from build123d import *

# Parameters (mm, degrees)
EXTRUDE_1_DEPTH      = 2
SKETCH_2_W           = 7
SKETCH_2_H           = 24
SKETCH_2_W_2         = 6
SKETCH_2_H_2         = 23
EXTRUDE_2_DEPTH      = 2
SCALE_1_SCALE        = 3.5
SKETCH_4_W           = 15
SKETCH_4_H           = 100
EXTRUDE_3_DEPTH      = 100
EXTRUDE_3_DEPTH_BACK = 107
SKETCH_5_W           = 116.879299814
SKETCH_5_H           = 13.538789425
EXTRUDE_4_DEPTH      = 207
SKETCH_6_W           = 116.879299814
SKETCH_6_H           = 12
EXTRUDE_5_DEPTH      = 100
EXTRUDE_9_DEPTH      = 25
CUT_EXTRUDE_7_DEPTH  = 20
EXTRUDE_10_DEPTH     = 207
SKETCH_17_R          = 3
CUT_EXTRUDE_8_DEPTH  = 6
SKETCH_22_R          = 1.052884015
CUT_EXTRUDE_9_DEPTH  = 209.5
SKETCH_23_R          = 3.020401844
CUT_EXTRUDE_10_DEPTH = 10
SKETCH_25_R          = 1.39267654
CUT_EXTRUDE_11_DEPTH = 10


with BuildPart() as part:
    # 草图1 → 凸台-拉伸1 (new body)
    with BuildSketch(Plane.XY):
        with BuildLine():
            Line((20, -3.5), (-20, -3.5))
            ThreePointArc((-20, -3.5), (-23.5, 0), (-20, 3.5))
            Line((-20, 3.5), (20, 3.5))
            ThreePointArc((20, 3.5), (23.5, 0), (20, -3.5))
        make_face()
        with BuildLine():
            Line((20, -3), (-20, -3))
            ThreePointArc((-20, -3), (-23, 0), (-20, 3))
            Line((-20, 3), (20, 3))
            ThreePointArc((20, 3), (23, 0), (20, -3))
        make_face(mode=Mode.SUBTRACT)
    extrude(amount=EXTRUDE_1_DEPTH)

    # 草图2 → 凸台-拉伸2 (add)
    with BuildSketch(Plane.XY.offset(2)):
        with Locations((0, 15.5)):
            Rectangle(SKETCH_2_W, SKETCH_2_H)
        with Locations((0, 15.5)):
            Rectangle(SKETCH_2_W_2, SKETCH_2_H_2, mode=Mode.SUBTRACT)
    extrude(amount=-EXTRUDE_2_DEPTH)


with BuildPart() as part_1:
    # 缩放比例1: scaled about (0, 5.797269405, 1)
    add(part.part.scale(SCALE_1_SCALE).moved(Location((0, -14.493173513, -2.5))))

    # 草图4 → 凸台-拉伸3 (add, two sides)
    with BuildSketch(Plane.XY.offset(4.5)) as extrude_3_sk:
        with Locations((62.5, -76.743173512)):
            Rectangle(SKETCH_4_W, SKETCH_4_H)
        with BuildLine():
            Line((-82.25, -14.493173512), (-82.25, -126.743173512))
            Line((-82.25, -126.743173512), (-61.879299814, -126.743173512))
            Line((-61.879299814, -126.743173512), (-61.879299814, -26.743173512))
            Line((-61.879299814, -26.743173512), (-70, -26.743173512))
            ThreePointArc((-70, -26.743173512), (-78.66205807, -23.155231582), (-82.25, -14.493173512))
        make_face()
    extrude(amount=EXTRUDE_3_DEPTH)
    extrude(extrude_3_sk.sketch, amount=-EXTRUDE_3_DEPTH_BACK)

    # 草图5 → 凸台-拉伸4 (add)
    with BuildSketch(Plane.XY.offset(104.5)):
        with Locations((-3.439649907, -119.9737788)):
            Rectangle(SKETCH_5_W, SKETCH_5_H)
    extrude(amount=-EXTRUDE_4_DEPTH)

    # 草图6 → 凸台-拉伸5 (add)
    with BuildSketch(Plane(origin=(0, -26.743173512, 0), x_dir=(1, 0, 0), z_dir=(0, 1, 0))):
        with Locations((-3.439649907, 96.5)):
            Rectangle(SKETCH_6_W, SKETCH_6_H)
        with Locations((-3.439649907, -98.5)):
            Rectangle(SKETCH_6_W, SKETCH_6_H)
    extrude(amount=-EXTRUDE_5_DEPTH)

    # 草图13 → 凸台-拉伸9 (add)
    with BuildSketch(Plane(origin=(0, -26.743173512, 0), x_dir=(1, 0, 0), z_dir=(0, 1, 0))):
        Polygon((-61.879299814, 17.670485576), (70, 17.670485576), (70, 26.332926598), (-61.879299814, 26.332926598), (-70, 26.332926598), (-70, 17.670485576), align=None)
    extrude(amount=EXTRUDE_9_DEPTH)

    # 草图15 → 切除-拉伸7 (cut)
    with BuildSketch(Plane(origin=(0, 0, -26.332926598), x_dir=(-1, 0, 0), z_dir=(0, 0, -1))):
        Polygon((-68, -24.743173512), (-55, -24.743173512), (61.879299814, -24.743173512), (68, -24.743173512), (68, -3.743173512), (-68, -3.743173512), align=None)
    extrude(amount=-CUT_EXTRUDE_7_DEPTH, mode=Mode.SUBTRACT)

    # 草图16 → 凸台-拉伸10 (add)
    with BuildSketch(Plane(origin=(0, 0, -102.5), x_dir=(-1, 0, 0), z_dir=(0, 0, -1))):
        Polygon((70, 2.916238078), (70, -10.049559482), (70, -26.598724572), (70, -27.524233973), (82.25, -27.524233973), (82.25, -25.898140615), (82.262032783, 0), (82.262032783, 2.916238078), align=None)
    extrude(amount=-EXTRUDE_10_DEPTH)

    # 草图17 → 切除-拉伸8 (cut)
    with BuildSketch(Plane.ZY.offset(82.25)):
        with Locations((100.503767222, -63.454563981)):
            Circle(SKETCH_17_R)
        with Locations((0.185055836, -23.454563981)):
            Circle(SKETCH_17_R)
        with Locations((-98.502426721, -63.454563981)):
            Circle(SKETCH_17_R)
        with Locations((0.816253539, -103.454563981)):
            Circle(SKETCH_17_R)
    extrude(amount=-CUT_EXTRUDE_8_DEPTH, mode=Mode.SUBTRACT)

    # 草图22 → 切除-拉伸9 (cut, through all)
    with BuildSketch(Plane.XZ.offset(126.743173512)):
        with Locations((0, 12.678619429)):
            Circle(SKETCH_22_R)
    extrude(amount=-CUT_EXTRUDE_9_DEPTH, mode=Mode.SUBTRACT)

    # 草图23 → 切除-拉伸10 (cut)
    with BuildSketch(Plane.XY.offset(104.5)):
        with Locations((-5.57826907, -64.954384087)):
            Circle(SKETCH_23_R)
    extrude(amount=-CUT_EXTRUDE_10_DEPTH, mode=Mode.SUBTRACT)

    # 草图25 → 切除-拉伸11 (cut)
    with BuildSketch(Plane(origin=(0, 0, -102.5), x_dir=(-1, 0, 0), z_dir=(0, 0, -1))):
        with Locations((-36.937867187, -51.815580574)):
            Circle(SKETCH_25_R)
        with Locations((-4.301261441, -21.564928261)):
            Circle(SKETCH_25_R)
        with Locations((38.214874816, -34.703731774)):
            Circle(SKETCH_25_R)
        with Locations((48.094405328, -78.0931876)):
            Circle(SKETCH_25_R)
        with Locations((15.457799582, -108.343839913)):
            Circle(SKETCH_25_R)
        with Locations((-27.058336676, -95.2050364)):
            Circle(SKETCH_25_R)
    extrude(amount=-CUT_EXTRUDE_11_DEPTH, mode=Mode.SUBTRACT)


solid = part_1.part
Geometry check sheet. Reference: the model listing, model coordinates, mm. A direction names the side the tool comes from. Give positions to 0.01 mm unless a question says otherwise; leave off trailing zeros. Order: outer loops, then holes, each group sorted by start corner. A loop starts at its lowest first (then second) coordinate and runs counter-clockwise, first axis right, second up.
1) Tool access check on faces 4 (the flat face through (-76.25, -63, -99)), 5 (the flat face through (-66, -26.743, -10)), 6 (the flat face through (12.25, 39, 1)), 7 (the cylindrical face through (80.5, -14.3, 1)). Record the directions out of +Z, -Z, +X, -X, +Y, -Y that give a thin tool (end or side, any length) a straight path to the whole face; none if there is none.
Results are:
face 4: -X
face 5: +X, +Y
face 6: +Z, -Z, +X, +Y
face 7: +Z, -Z
2) Cross-section at B-B (y = -85.5). Record the boundary of the cut face in (x, z).
Results are:
outline: (-82.25, -102.5) - (70, -102.5) - (70, 104.5) - (-82.25, 104.5) - close; hole (-61.88, -90.5) - (55, -90.5) - (55, 92.5) - (-61.88, 92.5) - close
3) Cross-section at A-A (x = 65). Record the boundary of the cut face in (y, z).
Results are:
outline: (-126.74, -102.5) - (-26.74, -102.5) - (-26.74, -26.33) - (-24.74, -26.33) - (-24.74, -17.67) - (-26.74, -17.67) - (-26.74, -2.5) - (-24.99, -2.5) - (-24.99, 4.5) - (-26.74, 4.5) - (-26.74, 104.5) - (-126.74, 104.5) - close; (-3.99, -2.5) - (-2.24, -2.5) - (-2.24, 4.5) - (-3.99, 4.5) - close; (-3.74, -26.33) - (-1.74, -26.33) - (-1.74, -17.67) - (-3.74, -17.67) - close
4) Cross-section at C-C (z = -48). Record the boundary of the cut face in (x, y).
Results are:
outline: (-82.26, 0) - (-82.25, -25.9) - (-82.25, -126.74) - (70, -126.74) - (70, -26.74) - (55, -26.74) - (55, -113.2) - (-61.88, -113.2) - (-61.88, -26.74) - (-70, -26.74) - (-70, 2.92) - (-82.26, 2.92) - close
5) Cross-section at D-D (x = 44). Record the boundary of the cut face in (y, z).
Results are:
outline: (-126.74, -102.5) - (-26.74, -102.5) - (-26.74, -90.5) - (-113.2, -90.5) - (-113.2, 92.5) - (-26.74, 92.5) - (-26.74, 104.5) - (-126.74, 104.5) - close; (-26.74, -26.33) - (-24.74, -26.33) - (-24.74, -17.67) - (-26.74, -17.67) - close; (-26.74, -2.5) - (-24.99, -2.5) - (-24.99, 4.5) - (-26.74, 4.5) - close; (-3.99, -2.5) - (-2.24, -2.5) - (-2.24, 4.5) - (-3.99, 4.5) - close; (-3.74, -26.33) - (-1.74, -26.33) - (-1.74, -17.67) - (-3.74, -17.67) - close
6) Draft check along X on faces 1 (the flat face through (-4, -69, -90.5)), 2 (the flat face through (-76.25, -103, 1)), 3 (the flat face through (5, -26.743, -93)). Enter one of: released by +X, released by -X, zero draft, split by the parting line, or undercut.
Results are:
face 1: undercut
face 2: released by -X
face 3: zero draft
7) Gauge pin test, flat ends, axial feed: pin 1 (4.5 mm diameter, centred on y = -15.5, z = -21, fed in from +X); pin 2 (10 mm diameter, centred on x = -74, z = -26, fed in from +Y); pin 3 (5 mm diameter, centred on x = 25, z = 67.5, fed in from +Y). Record the tip position at first contact, or that the pin passes through.
Results are:
pin 1: stops at x = 70
pin 2: stops at y = 2.92
pin 3: stops at y = -113.2
8) Material ranges on probe 1 along X at (y, z) = (-61.5, 30.5); probe 2 along Z at (x, y) = (42.5, -71); probe 3 along Y at (x, z) = (-18, -15), recorded low to high.
Results are:
probe 1: x = -82.25 to -61.88, 55 to 70
probe 2: z = -102.5 to -90.5, 92.5 to 104.5
probe 3: y = -126.74 to -113.2
